The listing builds one solid part. Answer for the finished solid, in the listing's coordinates (mm). Face numbers are marked on the shaded views. A direction names the side the tool comes from. Round coordinates to 2 decimals unless told otherwise and drop trailing zeros. Order: outer loops, then holes, each group sorted by start corner. A loop starts at its lowest first (then second) coordinate and runs counter-clockwise, first axis right, second up. Notation, with made-up numbers: (-19, 1.25) -> (23, 1.25) arc R20 cw to (23, 6.25) -> close; hole circle Ø4 at (81.5, 1). An arc over 180 degrees is marked (long way). Answer in a Markdown table with one row per item. Add a question column.
```python
from build123d import *

# Parameters (mm, degrees)
SKETCH1_R           = 3.45
SKETCH1_R_2         = 2.1
BOSS_EXTRUDE1_DEPTH = 5
SKETCH2_R           = 1.1
BOSS_EXTRUDE2_DEPTH = 2


with BuildPart() as part:
    # Sketch1 → Boss-Extrude1 (new body)
    with BuildSketch(Plane(origin=(0, 0, 0), x_dir=(1, 0, 0), z_dir=(0, 1, 0))):
        Circle(SKETCH1_R)
        Circle(SKETCH1_R_2, mode=Mode.SUBTRACT)
    extrude(amount=BOSS_EXTRUDE1_DEPTH)

    # Sketch2 → Boss-Extrude2 (add)
    with BuildSketch(Plane(origin=(0, 5, 0), x_dir=(1, 0, 0), z_dir=(0, 1, 0))):
        with BuildLine():
            Line((-3.282257873, 1.215229712), (-0.937787964, 7.547493269))
            ThreePointArc((-0.937787964, 7.547493269), (0, 8.200284779), (0.937787964, 7.547493269))
            Line((0.937787964, 7.547493269), (3.282257873, 1.215229712))
            ThreePointArc((3.282257873, 1.215229712), (3.5, 0), (3.282257873, -1.215229712))
            Line((3.282257873, -1.215229712), (0.937787964, -7.547493269))
            ThreePointArc((0.937787964, -7.547493269), (0, -8.200284779), (-0.937787964, -7.547493269))
            Line((-0.937787964, -7.547493269), (-3.282257873, -1.215229712))
            ThreePointArc((-3.282257873, -1.215229712), (-3.5, 0), (-3.282257873, 1.215229712))
        make_face()
        with Locations((0, -5.6)):
            Circle(SKETCH2_R, mode=Mode.SUBTRACT)
        with Locations((0, 5.6)):
            Circle(SKETCH2_R, mode=Mode.SUBTRACT)
    extrude(amount=BOSS_EXTRUDE2_DEPTH)


solid = part.part
```
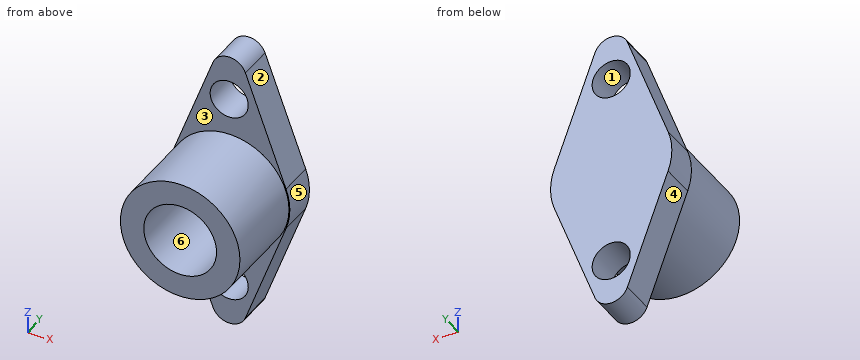
Item 1: Flat-ended cylindrical pins translate along their axes: P1, Ø2.5, axis at x = 0, z = -5.6, coming from the -Y side; P2, Ø3, axis at x = -0.5, y = 3, coming from the +Z side; P3, Ø3.5, axis at x = 0, z = 5.6, coming from the +Y side; P4, Ø2, axis at y = 6, z = 5, coming from the +X side. Find the tip coordinate at first contact, or state that the pin passes through.
Item 2: The part is cut by section D-D, the plane z = 0. Give the vertices of the cut face in (x, y), and give its area (3 significant figures).
Item 3: For a pull along Z with two mould halves and no side action, classify the marked faces 1, 2, 3 and 4 as released by +Z, released by -Z, zero draft, split by the parting line, or undercut.
Item 4: The part is cut by section A-A, the plane x = 0. Give the vertices of the cut face in (y, z).
Item 5: A tool of negligible diameter and unlimited length cuts with its end or side. For the marked faces 5 and 6, from which of +Z, -Z, +X, -X, +Y, -Y can it reach the whole face along a straight path? Write none if from no direction.
Item 6: The part is cut by section B-B, the plane y = 6.25. Give the vertices of the cut face in (x, z).
Item 7: The part is cut by section C-C, the plane z = -5.6. Give the vertices of the cut face in (x, y), and give its area (3 significant figures).
Item 8: Find the intervals of material crossed by probe 1 along X at (y, z) = (2.65, 0); probe 2 along Z at (x, y) = (0.5, 5.25), in increasing order. Write a range as [from, to].
Resolved:
| question | item | result |
|---|---|---|
| 1 | P1 | y = 5 |
| 1 | P2 | z = 3.45 |
| 1 | P3 | y = 7 |
| 1 | P4 | x = 2.25 |
| 2 | outline | (-3.5, 5) -> (-3.45, 5) -> (-3.45, 0) -> (-2.1, 0) -> (-2.1, 5) -> (2.1, 5) -> (2.1, 0) -> (3.45, 0) -> (3.45, 5) -> (3.5, 5) -> (3.5, 7) -> (-3.5, 7) -> close |
| 2 | area | 27.5 mm2 |
| 3 | face 1 | undercut |
| 3 | face 2 | released by +Z |
| 3 | face 3 | zero draft |
| 3 | face 4 | released by -Z |
| 4 | outline | (0, -3.45) -> (5, -3.45) -> (5, -4.5) -> (7, -4.5) -> (7, 4.5) -> (5, 4.5) -> (5, 3.45) -> (0, 3.45) -> (0, 2.1) -> (5, 2.1) -> (5, -2.1) -> (0, -2.1) -> close; (5, -8.2) -> (7, -8.2) -> (7, -6.7) -> (5, -6.7) -> close; (5, 6.7) -> (7, 6.7) -> (7, 8.2) -> (5, 8.2) -> close |
| 5 | face 5 | +X, +Y, -Y |
| 5 | face 6 | -Y |
| 6 | outline | (-3.28, -1.22) -> (-0.94, -7.55) arc R1 ccw to (0.94, -7.55) -> (3.28, -1.22) arc R3.5 ccw to (3.28, 1.22) -> (0.94, 7.55) arc R1 ccw to (-0.94, 7.55) -> (-3.28, 1.22) arc R3.5 ccw to start; hole circle Ø2.2 at (0, -5.6); hole circle Ø2.2 at (0, 5.6) |
| 7 | outline | (-1.66, 5) -> (-1.1, 5) -> (-1.1, 7) -> (-1.66, 7) -> close; (1.1, 5) -> (1.66, 5) -> (1.66, 7) -> (1.1, 7) -> close |
| 7 | area | 2.24 mm2 |
| 8 | probe 1 | [-3.45, -2.1], [2.1, 3.45] |
| 8 | probe 2 | [-8.07, -6.58], [-4.62, 4.62], [6.58, 8.07] |
